Source: CAD feature listing. Evaluate the final solid. Frame: model axes, mm. A direction names the side the tool comes from. Give positions to 0.01 mm unless a question says otherwise; leave off trailing zeros. Order: outer loops, then holes, each group sorted by start corner. A loop starts at its lowest first (then second) coordinate and runs counter-clockwise, first axis right, second up.
1) Section B-B, the plane z = 10.75. Return loops of the section in (x, y), plus the area to 3 significant figures.
2) Section C-C, the plane x = 0. Return loops of the section in (y, z).
3) Section A-A, the plane x = -11. Return loops of the section in (y, z), plus the area to 3 significant figures.
4) First-contact query: P1, Ø2.5, axis at x = -11.51, z = 11.51, coming from the +Y side; P2, Ø10, axis at x = 11.5, y = -6.5, coming from the -Z side; P3, Ø12, axis at x = 0.5, y = -9.5, coming from the -Z side; P4, Ø3, axis at y = -9, z = -8.5, coming from the +X side. Flat tips, straight axial feed; report the tip coordinate or a pass-through.
5) Section D-D, the plane z = 4.25. Return loops of the section in (x, y), plus the area to 3 significant figures.
6) Material intervals for line 1 (Y direction, x = 10.75, z = 2.5); line 2 (Y direction, x = 7.5, z = -12.5); line 3 (Z direction, x = 8, y = 4.5), sorted ascending.
7) Access query for faces 5 (the face through (-1.89, -6.39, -8.49)), 6 (the face through (-2.75, 11.33, 12.4)), 7 (the face through (-13.5, 2.06, 13.46)). Directions: +Z, -Z, +X, -X, +Y, -Y. A direction counts if a zero-diameter tool reaches every point of the face in a straight line with its end or side. Return the directions, or none.
8) Draft query along Z for faces 1 (the face through (10.629, 2.004, -12.882)), 2 (the face through (-7, 0, -7)), 3 (the face through (0, 2, 14.224)), 4 (the face through (-11.294, 2.004, -13.124)). Return one class per face: released by +Z, released by -Z, zero draft, split by the parting line, or undercut.
```python
from build123d import *

# Parameters (mm, degrees)
SKETCH1_W                 = 28.448
SKETCH1_H                 = 28.448
BOSS_EXTRUDE1_DEPTH       = 4.064
SKETCH2_R                 = 12.7
BOSS_EXTRUDE2_DEPTH       = 14.732
SKETCH3_R                 = 8.6995
BOSS_EXTRUDE3_DEPTH       = 12.954
F_4_CLEARANCE_HOLE1_D     = 3.2639
F_4_CLEARANCE_HOLE1_DEPTH = 7.62
F_4_CLEARANCE_HOLE1_TIP   = 0.980574487
FILLET1_R                 = 2.54


with BuildPart() as part:
    # Sketch1 → Boss-Extrude1 (new body)
    with BuildSketch(Plane(origin=(0, 0, 0), x_dir=(1, 0, 0), z_dir=(0, 1, 0))):
        Rectangle(SKETCH1_W, SKETCH1_H)
    extrude(amount=BOSS_EXTRUDE1_DEPTH)

    # Sketch2 → Boss-Extrude2 (add)
    with BuildSketch(Plane(origin=(0, 4.064, 0), x_dir=(1, 0, 0), z_dir=(0, 1, 0))):
        Circle(SKETCH2_R)
    extrude(amount=BOSS_EXTRUDE2_DEPTH)

    # Sketch3 → Boss-Extrude3 (add)
    with BuildSketch(Plane.XZ):
        Circle(SKETCH3_R)
    extrude(amount=BOSS_EXTRUDE3_DEPTH)

    # #4 Clearance Hole1
    with Locations(Plane(origin=(0, 4.064, 0), x_dir=(1, 0, 0), z_dir=(0, 1, 0))):
        with Locations((-11.5062, -11.5062), (11.5062, 11.5062), (-11.5062, 11.5062), (11.5062, -11.5062)):
            Hole(F_4_CLEARANCE_HOLE1_D / 2, depth=F_4_CLEARANCE_HOLE1_DEPTH)
            with Locations((0, 0, -(F_4_CLEARANCE_HOLE1_DEPTH + F_4_CLEARANCE_HOLE1_TIP / 2))):  # 118° drill point
                Cone(0, F_4_CLEARANCE_HOLE1_D / 2, F_4_CLEARANCE_HOLE1_TIP, mode=Mode.SUBTRACT)

    # Fillet1
    fillet1_edges = [part.edges().sort_by_distance(p)[0] for p in [
        (14.224, 2.032, 14.224),
        (-14.224, 2.032, 14.224),
        (-14.224, 2.032, -14.224),
        (14.224, 2.032, -14.224),
    ]]
    fillet(fillet1_edges, radius=FILLET1_R)


solid = part.part
```
From the geometry:
1. outline: (-14.22, 0) - (-12.95, 0) - (-12.95, 4.06) - (-14.22, 4.06) - close; (-10.06, 0) - (10.06, 0) - (10.06, 4.06) - (6.76, 4.06) - (6.76, 18.8) - (-6.76, 18.8) - (-6.76, 4.06) - (-10.06, 4.06) - close; (12.95, 0) - (14.22, 0) - (14.22, 4.06) - (12.95, 4.06) - close
1. area: 291 mm2
2. outline: (-12.95, -8.7) - (0, -8.7) - (0, -14.22) - (4.06, -14.22) - (4.06, -12.7) - (18.8, -12.7) - (18.8, 12.7) - (4.06, 12.7) - (4.06, 14.22) - (0, 14.22) - (0, 8.7) - (-12.95, 8.7) - close
3. outline: (0, -14.22) - (4.06, -14.22) - (4.06, -13.06) - (0, -13.06) - close; (0, -9.95) - (4.06, -9.95) - (4.06, -6.35) - (18.8, -6.35) - (18.8, 6.35) - (4.06, 6.35) - (4.06, 9.95) - (0, 9.95) - close; (0, 13.06) - (4.06, 13.06) - (4.06, 14.22) - (0, 14.22) - close
3. area: 277 mm2
4. P1: passes through
4. P2: stops at z = -5.78
4. P3: stops at z = -8.7
4. P4: stops at x = 5.17
5. outline: (-14.22, 0) - (-7.59, 0) - (-7.59, -12.95) - (7.59, -12.95) - (7.59, 0) - (14.22, 0) - (14.22, 4.06) - (11.97, 4.06) - (11.97, 18.8) - (-11.97, 18.8) - (-11.97, 4.06) - (-14.22, 4.06) - close
5. area: 665 mm2
6. line 1: y = 0 to 18.8
6. line 2: y = 0 to 4.06
6. line 3: z = -9.86 to 9.86
7. face 5: -Y
7. face 6: +Y
7. face 7: +Z, -X, +Y, -Y
8. face 1: undercut
8. face 2: zero draft
8. face 3: released by +Z
8. face 4: undercut
